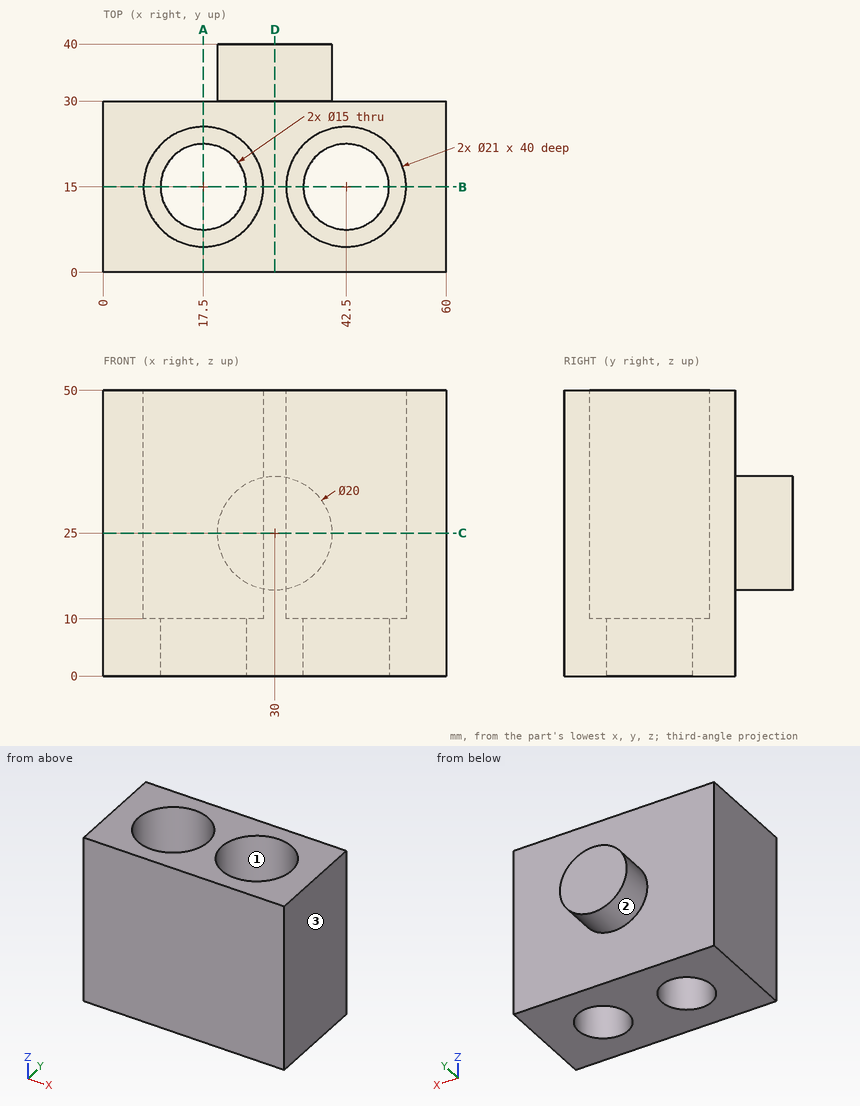
Design review of the part shown in the three views and the two pictorial views. Dimensions are in mm from the part's minimum x, y and z. A direction names the side the tool comes from. Give positions to 0.01 mm unless a question says otherwise; leave off trailing zeros. Loops run counter-clockwise (first coordinate to the right, second up) from the corner with the lowest first, then second, coordinate; pieces in that order, holes last. Notation, with made-up numbers: (66.25, 20.25) -> (84.25, 20.25) arc R33 cw to (84.25, 55.25) -> close; hole circle Ø2 at (59, 74.25). An arc over 180 degrees is marked (long way). One line per item, written item: value.
Q1. We need section B-B on y = 15. Give the boundary of the cut face in (x, z), and give its area (3 significant figures).
Numbers:
outline: (0, 0) -> (10, 0) -> (10, 10) -> (7, 10) -> (7, 50) -> (0, 50) -> close; (25, 0) -> (35, 0) -> (35, 10) -> (32, 10) -> (32, 50) -> (28, 50) -> (28, 10) -> (25, 10) -> close; (50, 0) -> (60, 0) -> (60, 50) -> (53, 50) -> (53, 10) -> (50, 10) -> close
area: 1,020 mm^2
Q2. For L1, parallel to Y at x = 42, z = 42; L2, parallel to Y at x = 17, z = 5; L3, parallel to X at y = 12.5, z = 11.5, list the stretches that pass through material, from the lowest coordinate up.
Numbers:
L1: y = 0 to 4.51, 25.49 to 30
L2: y = 0 to 7.52, 22.48 to 30
L3: x = 0 to 7.3, 27.7 to 32.3, 52.7 to 60
Q3. Machinability: for the marked faces 1, 2 and 3, which of the approach directions +Z, -Z, +X, -X, +Y, -Y give a long, thin tool a straight path to every point of the face, cutting with its end or side? Answer none if there is none.
Numbers:
face 1: +Z
face 2: +Y
face 3: +Z, -Z, +X, +Y, -Y
Q4. We need section C-C on z = 25. Give the boundary of the cut face in (x, y), and give its area (3 significant figures).
Numbers:
outline: (0, 0) -> (60, 0) -> (60, 30) -> (40, 30) -> (40, 40) -> (20, 40) -> (20, 30) -> (0, 30) -> close; hole circle Ø21 at (17.5, 15); hole circle Ø21 at (42.5, 15)
area: 1,310 mm^2
Q5. We need section D-D on x = 30. Give the boundary of the cut face in (y, z).
Numbers:
outline: (0, 0) -> (30, 0) -> (30, 15) -> (40, 15) -> (40, 35) -> (30, 35) -> (30, 50) -> (0, 50) -> close
Q6. We need section A-A on x = 17.5. Give the boundary of the cut face in (y, z).
Numbers:
outline: (0, 0) -> (7.5, 0) -> (7.5, 10) -> (4.5, 10) -> (4.5, 50) -> (0, 50) -> close; (22.5, 0) -> (30, 0) -> (30, 50) -> (25.5, 50) -> (25.5, 10) -> (22.5, 10) -> close
Q7. For pin 1 Ø10 at (x, y) = (17, 18.5) entering from +Z; pin 2 Ø12 at (x, y) = (20.5, 35) entering from +Z; pin 3 Ø12.5 at (x, y) = (17.5, 15) entering from -Z; pin 4 Ø5 at (x, z) = (37.5, 41.5) entering from +Y, all flat-tipped, find the tip position at first contact; note any pin that passes through.
Numbers:
pin 1: stops at z = 10
pin 2: stops at z = 50
pin 3: passes through
pin 4: stops at y = 30
